Autodesk Inventor part; units mm, degrees
ref_plane "Start plane" through (0, 0, -17.5) normal (0, 0, 1) x (1, 0, 0)
ref_plane "End plane" through (0, 0, 517.5) normal (0, 0, 1) x (1, 0, 0)
ref_plane "Work Plane4" through (107.5, 0, -17.5) normal (0, 0, -1) x (-1, 0, 0)
ref_plane "Start plane" through (0, 0, -17.5) normal (0, 0, 1) x (1, 0, 0)
ref_plane "End plane" through (0, 0, 517.5) normal (0, 0, 1) x (1, 0, 0)
sketch "Sketch" plane through (0, 0, 0) normal (0, 0, 1) x (1, 0, 0)
  line L0 (-17.5, -14.3) -> (-17.5, 14.3)
  line L1 (-14.3, 17.5) -> (14.3, 17.5)
  line L2 (17.5, 14.3) -> (17.5, -14.3)
  line L3 (14.3, -17.5) -> (-14.3, -17.5)
  arc A0 (-17.5, -14.3) -> (-14.3, -17.5) centre (-14.3, -14.3) ccw
  arc A1 (-14.3, 17.5) -> (-17.5, 14.3) centre (-14.3, 14.3) ccw
  arc A2 (17.5, 14.3) -> (14.3, 17.5) centre (14.3, 14.3) ccw
  arc A3 (14.3, -17.5) -> (17.5, -14.3) centre (14.3, -14.3) ccw
  arc A4 (-14.3, 15.9) -> (-15.9, 14.3) centre (-14.3, 14.3) ccw
  line L4 (-14.3, 15.9) -> (14.3, 15.9)
  arc A5 (15.9, 14.3) -> (14.3, 15.9) centre (14.3, 14.3) ccw
  line L5 (15.9, 14.3) -> (15.9, -14.3)
  arc A6 (14.3, -15.9) -> (15.9, -14.3) centre (14.3, -14.3) ccw
  line L6 (14.3, -15.9) -> (-14.3, -15.9)
  arc A7 (-15.9, -14.3) -> (-14.3, -15.9) centre (-14.3, -14.3) ccw
  line L7 (-15.9, -14.3) -> (-15.9, 14.3)
  line L8 (0, 25.4278) -> (0, -25.4278) construction
  line L9 (-25.4278, 0) -> (25.4278, 0) construction
  dimension "d7" = 3.2
  dimension "d10" = 35
  dimension "d11" = 35
  dimension "d12" = 1.6
  dimension "d15" = 17.5
  dimension "d16" = 17.5
extrude "Body" add sketch "Sketch" along normal up to surface (535 mm away) from surface at -17.5
sketch "Sketch3" plane through (0, 0, 0) normal (0, 0, 1) x (1, 0, 0)
  line L0 (0, 0) -> (10, 0)
ref_plane "Work Plane3" through (0, 0, 0) normal (0, -1, 0) x (1, 0, 0)
sketch "Sketch4" plane through (0, 0, 0) normal (0, -1, 0) x (1, 0, 0)
  line L0 (-2, -17.5) -> (12, -17.5)
  line L1 (-2, 517.5) -> (12, 517.5)
  dimension "d18" = 535
ref_plane "Work Plane4" through (107.5, 0, -17.5) normal (0, 0, -1) x (-1, 0, 0)
split "Split1" plane through (107.5, 0, -17.5) removes the side toward (0, 0, -1)
ref_plane "Work Plane5" through (0, -17.5, 517.5) normal (0, 0.7071, 0.7071) x (1, 0, 0)
split "Split2" plane through (0, -17.5, 517.5) removes the side toward (0, 0.7071, 0.7071)
ref_plane "Work Plane7" through (0, 800, 400) normal (0, -1, 0) x (1, 0, 0)
ref_plane "Work Plane8" through (0, 0, 400) normal (0, -1, 0) x (1, 0, 0)
ref_plane "Work Plane9" through (0, 400, 400) normal (0, -1, 0) x (1, 0, 0)
ref_plane "Work Plane10" through (0, 0, 100) normal (0, 1, 0) x (-1, 0, 0)
ref_plane "Work Plane11" through (0, 800, 100) normal (0, 1, 0) x (-1, 0, 0)
ref_plane "Work Plane12" through (0, 400, 100) normal (0, 1, 0) x (-1, 0, 0)
sketch "Sketch5" plane through (0, 400, 400) normal (0, -1, 0) x (1, 0, 0)
  arc A0 (-17.5, -14.3) -> (-14.3, -17.5) centre (-14.3, -14.3) ccw
  line L0 (-17.5, -14.3) -> (-17.5, 14.3)
  arc A1 (-14.3, 17.5) -> (-17.5, 14.3) centre (-14.3, 14.3) ccw
  line L1 (-14.3, 17.5) -> (14.3, 17.5)
  arc A2 (17.5, 14.3) -> (14.3, 17.5) centre (14.3, 14.3) ccw
  line L2 (17.5, 14.3) -> (17.5, -14.3)
  arc A3 (14.3, -17.5) -> (17.5, -14.3) centre (14.3, -14.3) ccw
  line L3 (14.3, -17.5) -> (-14.3, -17.5)
  arc A4 (-14.3, 15.9) -> (-15.9, 14.3) centre (-14.3, 14.3) ccw
  line L4 (-14.3, 15.9) -> (14.3, 15.9)
  arc A5 (15.9, 14.3) -> (14.3, 15.9) centre (14.3, 14.3) ccw
  line L5 (15.9, 14.3) -> (15.9, -14.3)
  arc A6 (14.3, -15.9) -> (15.9, -14.3) centre (14.3, -14.3) ccw
  line L6 (14.3, -15.9) -> (-14.3, -15.9)
  arc A7 (-15.9, -14.3) -> (-14.3, -15.9) centre (-14.3, -14.3) ccw
  line L7 (-15.9, -14.3) -> (-15.9, 14.3)
extrude "Extrusion2" cut sketch "Sketch5" along normal up to surface (800 mm away) from surface at -400 contours L0 A1 L1 A2 L2 A3 L3 A0 | L4 A5 L5 A6 L6 A7 L7 A4
sketch "Sketch6" plane through (0, 400, 100) normal (0, 1, 0) x (-1, 0, 0)
  arc A0 (-17.5, -14.3) -> (-14.3, -17.5) centre (-14.3, -14.3) ccw
  line L0 (-17.5, -14.3) -> (-17.5, 14.3)
  arc A1 (-14.3, 17.5) -> (-17.5, 14.3) centre (-14.3, 14.3) ccw
  line L1 (-14.3, 17.5) -> (14.3, 17.5)
  arc A2 (17.5, 14.3) -> (14.3, 17.5) centre (14.3, 14.3) ccw
  line L2 (17.5, 14.3) -> (17.5, -14.3)
  arc A3 (14.3, -17.5) -> (17.5, -14.3) centre (14.3, -14.3) ccw
  line L3 (14.3, -17.5) -> (-14.3, -17.5)
  arc A4 (-14.3, 15.9) -> (-15.9, 14.3) centre (-14.3, 14.3) ccw
  line L4 (-14.3, 15.9) -> (14.3, 15.9)
  arc A5 (15.9, 14.3) -> (14.3, 15.9) centre (14.3, 14.3) ccw
  line L5 (15.9, 14.3) -> (15.9, -14.3)
  arc A6 (14.3, -15.9) -> (15.9, -14.3) centre (14.3, -14.3) ccw
  line L6 (14.3, -15.9) -> (-14.3, -15.9)
  arc A7 (-15.9, -14.3) -> (-14.3, -15.9) centre (-14.3, -14.3) ccw
  line L7 (-15.9, -14.3) -> (-15.9, 14.3)
extrude "Extrusion3" cut sketch "Sketch6" along normal up to surface (800 mm away) from surface at -400 contours L0 A1 L1 A2 L2 A3 L3 A0 | L4 A5 L5 A6 L6 A7 L7 A4
ref_plane "Work Plane13" through (0, -17.5, -17.5) normal (0, 0.7071, -0.7071) x (1, 0, 0)
split "Split4" plane through (0, -17.5, -17.5) removes the side toward (0, 0.7071, -0.7071)
equation "\"d7\" = G_IR"
equation "\"d10\" = G_H"
equation "\"d11\" = G_W"
equation "\"d12\" = G_T"
equation "\"d15\" = 0.5 * d10"
equation "\"d16\" = 0.5 * d11"
equation "\"d3\" = G_L"
equation "\"G_W\" = 35"
equation "\"G_H\" = 35"
equation "\"G_T\" = 1.6"
equation "\"G_IR\" = 3.2"
equation "\"G_L\" = d18"
equation "\"G_OFFSET_START\" = 17.5"
equation "\"G_OFFSET_END\" = 17.5"
equation "\"d13\" = -G_OFFSET_START"
equation "\"d14\" = G_OFFSET_END + B_L"
properties part number "AS 1163 - C350L0 35x35x1.6 SHS - 535" material "Steel, Mild"
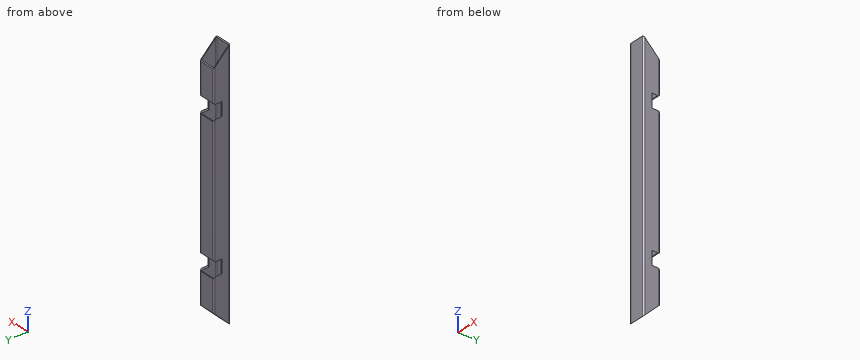
For this review, take the finished solid that the model builds, in its own axes (mm). Coordinates: 2 decimals unless noted, no trailing zeros. Write each loop counter-clockwise with the first axis right and the second up, starting at its lowest first coordinate (ties: lowest second). Pieces come first, ordered by that corner, then holes. Notation, with made-up numbers: (29, 58.25) -> (45, 58.25) arc R33 cw to (45, 89.25) -> close; hole circle Ø3 at (-35, 30). An arc over 180 degrees is marked (long way). Write each question's results on one line, items separated by ' | '. Start each with the question number.
1) Consider section B-B (z = 313.5). Write out the cut boundary in (x, y), plus the area to 3 significant figures.
2) Wall thickness on L1, parallel to X at y = 8, z = 239; L2, parallel to Y at x = -13, z = 389: over which ranges is each line inside the solid? List them lowest first. Write a range as [from, to].
3) Consider section A-A (y = 4.5). Write out the cut boundary in (x, z), plus the area to 3 significant figures.
4) Consider section D-D (z = 396.5). Write out the cut boundary in (x, y), plus the area to 3 significant figures.
5) Consider section C-C (x = 10). Write out the cut boundary in (y, z), plus the area to 3 significant figures.
6) Insertion check: pin 1 (0.5 mm diameter, centred on x = -16.5, z = 106.5, fed in from +Y); pin 2 (0.5 mm diameter, centred on x = -3, y = 17, fed in from -Z); pin 3 (0.5 mm diameter, centred on x = 0.5, y = 17, fed in from +Z); pin 4 (10 mm diameter, centred on x = -8, y = 7.5, fed in from -Z). Each pin has a flat end and moves straight along its axis. Give the tip position at first contact, or say it passes through.
Geometry says:
1) outline: (-17.5, -14.3) arc R3.2 ccw to (-14.3, -17.5) -> (14.3, -17.5) arc R3.2 ccw to (17.5, -14.3) -> (17.5, 14.3) arc R3.2 ccw to (14.3, 17.5) -> (-14.3, 17.5) arc R3.2 ccw to (-17.5, 14.3) -> close; hole (-15.9, -14.3) arc R1.6 ccw to (-14.3, -15.9) -> (14.3, -15.9) arc R1.6 ccw to (15.9, -14.3) -> (15.9, 14.3) arc R1.6 ccw to (14.3, 15.9) -> (-14.3, 15.9) arc R1.6 ccw to (-15.9, 14.3) -> close | area: 207 mm^2
2) L1: [-17.5, -15.9], [15.9, 17.5] | L2: [-17.5, -15.9]
3) outline: (-17.5, 4.5) -> (-15.9, 4.5) -> (-15.9, 82.93) arc R3.2 cw to (-17.5, 85.7) -> close; (-17.5, 114.3) arc R3.2 cw to (-15.9, 117.07) -> (-15.9, 382.93) arc R3.2 cw to (-17.5, 385.7) -> close; (-17.5, 414.3) arc R3.2 cw to (-15.9, 417.07) -> (-15.9, 495.5) -> (-17.5, 495.5) -> close; (15.9, 4.5) -> (17.5, 4.5) -> (17.5, 85.7) arc R3.2 cw to (15.9, 82.93) -> close; (15.9, 117.07) arc R3.2 cw to (17.5, 114.3) -> (17.5, 385.7) arc R3.2 cw to (15.9, 382.93) -> close; (15.9, 417.07) arc R3.2 cw to (17.5, 414.3) -> (17.5, 495.5) -> (15.9, 495.5) -> close | area: 1,360 mm^2
4) outline: (-17.5, -14.3) arc R3.2 ccw to (-14.3, -17.5) -> (14.3, -17.5) arc R3.2 ccw to (17.5, -14.3) -> (17.5, 0) -> (15.9, 0) -> (15.9, -14.3) arc R1.6 cw to (14.3, -15.9) -> (-14.3, -15.9) arc R1.6 cw to (-15.9, -14.3) -> (-15.9, 0) -> (-17.5, 0) -> close | area: 104 mm^2
5) outline: (-17.5, -17.5) -> (-15.9, -15.9) -> (-15.9, 515.9) -> (-17.5, 517.5) -> close; (15.9, 15.9) -> (17.5, 17.5) -> (17.5, 82.5) -> (15.9, 82.5) -> close; (15.9, 117.5) -> (17.5, 117.5) -> (17.5, 382.5) -> (15.9, 382.5) -> close; (15.9, 417.5) -> (17.5, 417.5) -> (17.5, 482.5) -> (15.9, 484.1) -> close | area: 1,490 mm^2
6) pin 1: y = 0 | pin 2: z = 16.75 | pin 3: z = 483.25 | pin 4: through
